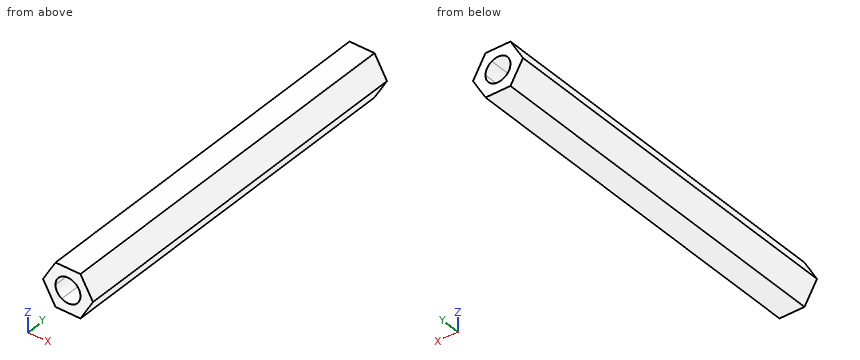
```python
from build123d import *

# Parameters (mm, degrees)
EXTRUDE_1_DEPTH = 60


with BuildPart() as part:
    # 草图1 → 凸台-拉伸1 (new body)
    with BuildSketch(Plane(origin=(0, 0, 0), x_dir=(1, 0, 0), z_dir=(0, 1, 0))):
        with BuildLine():
            Line((2.09823197, 4.329567776), (-1.90176803, 4.329567776))
            Line((-1.90176803, 4.329567776), (-0.90176803, 2.597516968))
            ThreePointArc((-0.90176803, 2.597516968), (1.09823197, 2.597516968), (2.09823197, 0.865466161))
            Line((2.09823197, 0.865466161), (4.09823197, 0.865466161))
            Line((4.09823197, 0.865466161), (2.09823197, 4.329567776))
        make_face()
        with BuildLine():
            Line((-0.90176803, 2.597516968), (-1.90176803, 4.329567776))
            Line((-1.90176803, 4.329567776), (-3.90176803, 0.865466161))
            Line((-3.90176803, 0.865466161), (-1.90176803, 0.865466161))
            ThreePointArc((-1.90176803, 0.865466161), (-1.633818837, 1.865466161), (-0.90176803, 2.597516968))
        make_face()
        with BuildLine():
            Line((-1.90176803, 0.865466161), (-3.90176803, 0.865466161))
            Line((-3.90176803, 0.865466161), (-1.90176803, -2.598635455))
            Line((-1.90176803, -2.598635455), (2.09823197, -2.598635455))
            Line((2.09823197, -2.598635455), (1.09823197, -0.866584647))
            ThreePointArc((1.09823197, -0.866584647), (-0.90176803, -0.866584647), (-1.90176803, 0.865466161))
        make_face()
        with BuildLine():
            Line((2.09823197, -2.598635455), (4.09823197, 0.865466161))
            Line((4.09823197, 0.865466161), (2.09823197, 0.865466161))
            ThreePointArc((2.09823197, 0.865466161), (1.830282778, -0.134533839), (1.09823197, -0.866584647))
            Line((1.09823197, -0.866584647), (2.09823197, -2.598635455))
        make_face()
    extrude(amount=EXTRUDE_1_DEPTH)


solid = part.part
```
The listing builds one solid part. Answer for the finished solid, in the listing's coordinates (mm). Give positions to 0.01 mm unless a question says otherwise; leave off trailing zeros. Order: outer loops, then holes, each group sorted by start corner. A loop starts at its lowest first (then second) coordinate and runs counter-clockwise, first axis right, second up. Notation, with made-up numbers: (70.5, -9) - (74.5, -9) arc R33 cw to (74.5, 19) - close; hole circle Ø8 at (77, 0.5). An arc over 180 degrees is marked (long way). Answer in a Markdown table with one row per item. Add a question column.
Q1. The part is cut by section B-B (x = 0.5). Determine the outline of the cut face in (y, z), then the cut area to 3 significant figures.
Q2. Given P1, Ø2, axis at x = -2.5, y = 37.5, coming from the +Z side, flat-ended and moving along its own axis, determine where the tip first touches the part or whether it passes through.
Q3. The part is cut by section A-A (y = 6). Determine the outline of the cut face in (x, z).
Q4. The part is cut by section D-D (x = 3.5). Determine the outline of the cut face in (y, z), then the cut area to 3 significant figures.
Q5. Find the intervals of material crossed by line 1 along Z through (x, y) = (0.25, 36.5); line 2 along X through (y, z) = (12, -0.75); line 3 along Z through (x, y) = (-2.75, 17), in increasing order. Write a range as [from, to].
Q6. The part is cut by section C-C (z = 0.25). Determine the outline of the cut face in (x, y), then the cut area to 3 significant figures.
Determined:
| question | item | result |
|---|---|---|
| 1 | outline | (0, -4.33) - (60, -4.33) - (60, -2.82) - (0, -2.82) - close; (0, 1.09) - (60, 1.09) - (60, 2.6) - (0, 2.6) - close |
| 1 | area | 181 mm² |
| 2 | P1 | stops at z = 2.6 |
| 3 | outline | (-3.9, -0.87) - (-1.9, -4.33) - (2.1, -4.33) - (4.1, -0.87) - (2.1, 2.6) - (-1.9, 2.6) - close; hole circle Ø4 at (0.1, -0.87) |
| 4 | outline | (0, -1.9) - (60, -1.9) - (60, 0.17) - (0, 0.17) - close |
| 4 | area | 124 mm² |
| 5 | line 1 | z = [-4.33, -2.86], [1.13, 2.6] |
| 5 | line 2 | x = [-3.84, -1.9], [2.09, 4.03] |
| 5 | line 3 | z = [-2.86, 1.13] |
| 6 | outline | (-3.26, 0) - (-1.56, 0) - (-1.56, 60) - (-3.26, 60) - close; (1.76, 0) - (3.45, 0) - (3.45, 60) - (1.76, 60) - close |
| 6 | area | 204 mm² |
